Could you check a few things on this model? Use its own coordinates, in mm. Face numbers are marked on the shaded views. Coordinates: 2 decimals unless noted, no trailing zeros. Loops run counter-clockwise (first coordinate to the right, second up) from the corner with the lowest first, then second, coordinate; pieces in that order, holes last. Notation, with made-up numbers: (69, 48) -> (90, 48) arc R13 ccw to (90, 54) -> close; hole circle Ø11 at (34, 78). An arc over 180 degrees is marked (long way). One line per question, with ' | ' between items.
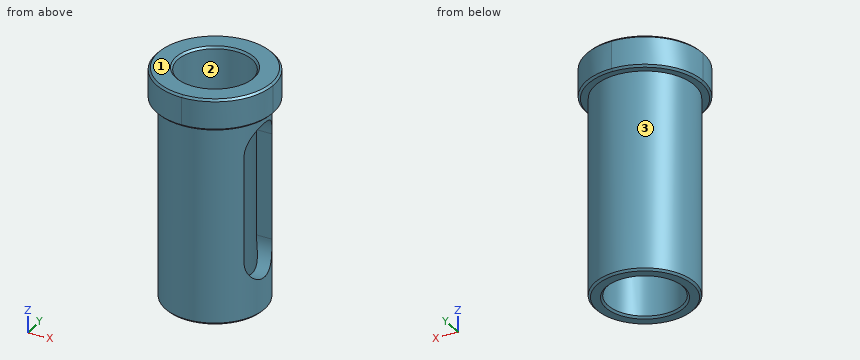
```python
from build123d import *

# Parameters (mm, degrees)
SCHIZZO1_W                   = 118
SCHIZZO1_H                   = 60
ESTRUSIONE_ESTRUSIONE1_DEPTH = 60
TAGLIO_ESTRUSIONE1_DEPTH     = 30
SCHIZZO3_W                   = 60
SCHIZZO3_H                   = 60
SCHIZZO3_R                   = 25.5
TAGLIO_ESTRUSIONE4_DEPTH     = 102
TAGLIO_ESTRUSIONE5_DEPTH     = 18
SCHIZZO5_R                   = 19
TAGLIO_ESTRUSIONE6_DEPTH     = 136.735036008
SMUSSO1_SIZE                 = 1
SMUSSO2_SIZE                 = 1
SMUSSO3_SIZE                 = 1
SMUSSO4_SIZE                 = 1
SMUSSO5_SIZE                 = 1


with BuildPart() as part:
    # Schizzo1 → Estrusione-Estrusione1 (new body)
    with BuildSketch(Plane(origin=(0, 0, 0), x_dir=(0, 0, -1), z_dir=(1, 0, 0))):
        Rectangle(SCHIZZO1_W, SCHIZZO1_H)
    extrude(amount=-ESTRUSIONE_ESTRUSIONE1_DEPTH)

    # Schizzo2 → Taglio-Estrusione1 (cut)
    with BuildSketch(Plane(origin=(0, 0, 0), x_dir=(0, 0, -1), z_dir=(1, 0, 0))):
        with BuildLine():
            Line((29, 12.534031414), (-25, 12.534031414))
            ThreePointArc((-25, 12.534031414), (-37.534031414, 0), (-25, -12.534031414))
            Line((-25, -12.534031414), (29, -12.534031414))
            ThreePointArc((29, -12.534031414), (41.534031414, 0), (29, 12.534031414))
        make_face()
    extrude(amount=-TAGLIO_ESTRUSIONE1_DEPTH, mode=Mode.SUBTRACT)

    # Schizzo3 → Taglio-Estrusione4 (cut)
    with BuildSketch(Plane(origin=(0, 0, -59), x_dir=(-1, 0, 0), z_dir=(0, 0, -1))):
        with Locations((30, 0)):
            Rectangle(SCHIZZO3_W, SCHIZZO3_H)
        with Locations((30, 0)):
            Circle(SCHIZZO3_R, mode=Mode.SUBTRACT)
    extrude(amount=-TAGLIO_ESTRUSIONE4_DEPTH, mode=Mode.SUBTRACT)

    # Schizzo4 → Taglio-Estrusione5 (cut)
    with BuildSketch(Plane.XY.offset(59)):
        with BuildLine():
            Line((-30, 30), (-60, 30))
            Line((-60, 30), (-60, 0))
            ThreePointArc((-60, 0), (-51.213203436, 21.213203436), (-30, 30))
        make_face()
        with BuildLine():
            Line((0, 30), (-30, 30))
            ThreePointArc((-30, 30), (-8.786796564, 21.213203436), (0, 0))
            Line((0, 0), (0, 30))
        make_face()
        with BuildLine():
            Line((0, -30), (0, 0))
            ThreePointArc((0, 0), (-8.786796564, -21.213203436), (-30, -30))
            Line((-30, -30), (0, -30))
        make_face()
        with BuildLine():
            ThreePointArc((-30, -30), (-51.213203436, -21.213203436), (-60, 0))
            Line((-60, 0), (-60, -30))
            Line((-60, -30), (-30, -30))
        make_face()
    extrude(amount=-TAGLIO_ESTRUSIONE5_DEPTH, mode=Mode.SUBTRACT)

    # Schizzo5 → Taglio-Estrusione6 (cut, through all)
    with BuildSketch(Plane(origin=(0, 0, -59), x_dir=(-1, 0, 0), z_dir=(0, 0, -1))):
        with Locations((30, 0)):
            Circle(SCHIZZO5_R)
    extrude(amount=-TAGLIO_ESTRUSIONE6_DEPTH, mode=Mode.SUBTRACT)

    # Smusso1
    smusso1_edges = [part.edges().sort_by_distance(p)[0] for p in [
        (-11, 0, -59),
    ]]
    chamfer(smusso1_edges, length=SMUSSO1_SIZE)

    # Smusso2
    smusso2_edges = [part.edges().sort_by_distance(p)[0] for p in [
        (-4.5, 0, -59),
    ]]
    chamfer(smusso2_edges, length=SMUSSO2_SIZE)

    # Smusso3
    smusso3_edges = [part.edges().sort_by_distance(p)[0] for p in [
        (-60, 0, 43),
    ]]
    chamfer(smusso3_edges, length=SMUSSO3_SIZE)

    # Smusso4
    smusso4_edges = [part.edges().sort_by_distance(p)[0] for p in [
        (-11, 0, 59),
    ]]
    chamfer(smusso4_edges, length=SMUSSO4_SIZE)

    # Smusso5
    smusso5_edges = [part.edges().sort_by_distance(p)[0] for p in [
        (-60, 0, 59),
    ]]
    chamfer(smusso5_edges, length=SMUSSO5_SIZE)


solid = part.part
```
Q1. Imagine slicing it at A-A on y = 6. Give the number of separate pieces and of enclosed holes in the cut face, plus the area to 3 significant figures.
Values follow:
separate pieces: 3 | enclosed holes: 0 | area: 1,220 mm2
Q2. Please list where these lines run through material, in increasing order: L1, parallel to Y at x = -30, z = -16; L2, parallel to Z at x = -21.5, y = 27; L3, parallel to X at y = -5, z = -42.5 (3 decimals). Write a range as [from, to].
Values follow:
L1: y = [-25.5, -19], [19, 25.5] | L2: z = [43, 59] | L3: x = [-55.005, -48.33], [-11.67, -4.995]
Q3. Imagine slicing it at B-B on z = 3. Write out the boundary of the cut face in (x, y), plus the area to 3 significant figures.
Values follow:
outline: (-15.72, -12.53) arc R19 cw (long way) to (-15.72, 12.53) -> (-7.79, 12.53) arc R25.5 ccw (long way) to (-7.79, -12.53) -> close | area: 735 mm2
Q4. Imagine slicing it at D-D on z = 28. Write out the boundary of the cut face in (x, y), plus the area to 3 significant figures.
Values follow:
outline: (-15.41, -12.17) arc R19 cw (long way) to (-15.41, 12.17) -> (-7.59, 12.17) arc R25.5 ccw (long way) to (-7.59, -12.17) -> close | area: 741 mm2
Q5. For pin 1 (6 mm diameter, centred on y = 0, z = -21.5, fed in from +X); pin 2 (4 mm diameter, centred on x = -10, z = 8.5, fed in from -Y); pin 3 (6 mm diameter, centred on x = -31.5, z = -11, fed in from +Y), each with a flat end and sliding along its axis, tell me the tip position at first contact or that it passes through.
Values follow:
pin 1: stops at x = -48.76 | pin 2: stops at y = -18.06 | pin 3: stops at y = 25.5
Q6. We'd pull the mould along X, two halves only. Please class the marked faces 1, 2 and 3: released by +X, released by -X, zero draft, split by the parting line, or undercut.
Values follow:
face 1: zero draft | face 2: undercut | face 3: split by the parting line
